```python
from build123d import *

# Parameters (mm, degrees)
SKETCH_1_R          = 1.6
SKETCH_1_R_2        = 2
EXTRUDE_1_DEPTH     = 3
CUT_EXTRUDE_1_DEPTH = 3
FILLET_1_R          = 50
FILLET_2_R          = 1


with BuildPart() as part:
    # ｽｹｯﾁ1 → ﾎﾞｽ - 押し出し1 (new body)
    with BuildSketch(Plane(origin=(0, 0, 0), x_dir=(1, 0, 0), z_dir=(0, 1, 0))):
        Polygon((0, 58.4), (35, 58.4), (35, 43.4), (57.5, 43.4), (57.5, 0), (0, 0), align=None)
        with Locations(Location((52.5, 7.4, 0), (0, 0, 270))):
            Circle(SKETCH_1_R, mode=Mode.SUBTRACT)
        with Locations(Location((52.5, 33.4, 0), (0, 0, 270))):
            Circle(SKETCH_1_R, mode=Mode.SUBTRACT)
        with Locations(Location((30, 53.4, 0), (0, 0, 270))):
            Circle(SKETCH_1_R_2, mode=Mode.SUBTRACT)
        with Locations(Location((5, 42.4, 0), (0, 0, 270))):
            Circle(SKETCH_1_R, mode=Mode.SUBTRACT)
        with Locations(Location((5, 6, 0), (0, 0, 90))):
            Circle(SKETCH_1_R, mode=Mode.SUBTRACT)
    extrude(amount=EXTRUDE_1_DEPTH)

    # ｽｹｯﾁ2 → ｶｯﾄ - 押し出し1 (cut)
    with BuildSketch(Plane(origin=(0, 3, 0), x_dir=(1, 0, 0), z_dir=(0, 1, 0))):
        Polygon((5, 58.4), (0, 58.4), (0, 43.4), align=None)
    extrude(amount=-CUT_EXTRUDE_1_DEPTH, mode=Mode.SUBTRACT)

    # ﾌｨﾚｯﾄ1
    fillet_1_edges = [part.edges().sort_by_distance(p)[0] for p in [
        (0, 1.5, -43.4),
    ]]
    fillet(fillet_1_edges, radius=FILLET_1_R)

    # ﾌｨﾚｯﾄ2
    fillet_2_edges = [part.edges().sort_by_distance(p)[0] for p in [
        (35, 1.5, -58.4),
        (35, 1.5, -43.4),
        (57.5, 1.5, -43.4),
        (57.5, 1.5, 0),
        (0, 1.5, 0),
        (5, 1.5, -58.4),
    ]]
    fillet(fillet_2_edges, radius=FILLET_2_R)


solid = part.part
```
Input: part model. Units: mm. Frame: model coordinates. A direction names the side the tool comes from. Give positions to 0.01 mm unless a question says otherwise; leave off trailing zeros. Loops run counter-clockwise (first coordinate to the right, second up) from the corner with the lowest first, then second, coordinate; pieces in that order, holes last. Notation, with made-up numbers: M -37.5,3.25 L 3.5,3.25 A38 cw 3.5,42.25 Z; hole C -6.5,22 d10. An arc over 180 degrees is marked long. Answer as CSV lines item,"result". Start each with the question number.
1. Section B-B on z = -33.4. Return loops of the section in (x, y).
2. Section A-A on x = 30. Return loops of the section in (y, z).
3. Pin query (flat end, axial travel): P1, Ø6, axis at x = 46, z = -31.5, coming from the -Y side; P2, Ø1.5, axis at y = 1, z = -52.5, coming from the +X side. Return the tip coordinate at first contact, or that it passes through.
4. Pull-direction query (X, two-part tool) for faces 3 (the face through (0.664, 1.479, -43.406)), 4 (the face through (29, 3, -30)), 5 (the face through (4.519, 1.479, -7.526)); classes: released by +X, released by -X, zero draft, split by the parting line, or undercut.
5. Section C-C on x = 52.5. Return loops of the section in (y, z).
6. Reachability of faces 1 (the face through (52.57, 1.48, -35)), 2 (the face through (35, 1, -51)) from +Z, -Z, +X, -X, +Y, -Y: full face, straight path, thin tool, end or side. Return the list, or none.
7. Line query: L1, parallel to X at y = 0.7, z = -7.4; L2, parallel to X at y = 1.8, z = -33.4; L3, parallel to X at y = 1.7, z = -6. Output: solid intervals per line, ascending.
8. Section D-D on y = 0.5. Return loops of the section in (x, z), plus the area to 3 significant figures.
Computed values:
1,outline,"M 0,0 L 50.9,0 L 50.9,3 L 0,3 Z; M 54.1,0 L 57.5,0 L 57.5,3 L 54.1,3 Z"
2,outline,"M 0,-58.4 L 3,-58.4 L 3,-55.4 L 0,-55.4 Z; M 0,-51.4 L 3,-51.4 L 3,0 L 0,0 Z"
3,P1,"stops at y = 0"
3,P2,"stops at x = 35"
4,face 3,"released by -X"
4,face 4,"zero draft"
4,face 5,"undercut"
5,outline,"M 0,-43.4 L 3,-43.4 L 3,-35 L 0,-35 Z; M 0,-31.8 L 3,-31.8 L 3,-9 L 0,-9 Z; M 0,-5.8 L 3,-5.8 L 3,0 L 0,0 Z"
6,face 1,"+Y, -Y"
6,face 2,"-Z, +X, +Y, -Y"
7,L1,"x = 0 to 4.23, 5.77 to 50.9, 54.1 to 57.5"
7,L2,"x = 0 to 50.9, 54.1 to 57.5"
7,L3,"x = 0 to 3.4, 6.6 to 51.73, 53.27 to 57.5"
8,outline,"M 0,-35.29 A50 ccw 2.57,-51.1 L 4.77,-57.72 A1 ccw 5.72,-58.4 L 34,-58.4 A1 ccw 35,-57.4 L 35,-44.4 A1 cw 36,-43.4 L 56.5,-43.4 A1 ccw 57.5,-42.4 L 57.5,-1 A1 ccw 56.5,0 L 1,0 A1 ccw 0,-1 Z; hole C 5,-42.4 d3.2; hole C 5,-6 d3.2; hole C 30,-53.4 d4; hole C 52.5,-33.4 d3.2; hole C 52.5,-7.4 d3.2"
8,area,"2,930 mm²"
